Read the model definition and answer for the solid it produces. Units are mm, in the model's axes. A direction names the side the tool comes from. Round coordinates to 2 decimals unless told otherwise and drop trailing zeros. Order: outer loops, then holes, each group sorted by start corner. A loop starts at its lowest first (then second) coordinate and runs counter-clockwise, first axis right, second up. Notation, with made-up numbers: (6.5, -16) -> (37.5, -16) arc R21 cw to (37.5, -7) -> close; hole circle Ø4 at (50.5, 45). An arc over 180 degrees is marked (long way). Use a Markdown table: item, result. Add a question column.
1. Section C-C, the plane z = -10 is taken. Give the vertices of the cut face in (x, y), then the cut area to 3 significant figures.
2. Given pin 1 (1 mm diameter, centred on x = 5.5, y = -23, fed in from +Z); pin 2 (1 mm diameter, centred on x = 36.5, z = -6, fed in from -Y); pin 3 (5 mm diameter, centred on x = 19.5, y = 2, fed in from -Z), each flat-ended and moving along its own axis, determine where each tip first touches the part or whether it passes through.
3. Consider L1, parallel to Z at x = 61, y = -42.5; L2, parallel to Z at x = 25.5, y = -21.5; L3, parallel to Y at x = 32, z = -8.25. Determine where each line is inside the solid, lowest interval first. Write a range as [from, to].
4. Section D-D, the plane x = 10 is taken. Give the vertices of the cut face in (y, z).
5. For faces 1 (the face through (24.716, -15.178, -6.261)), 2 (the face through (-21.634, 16.934, 7.915)), 3 (the face through (27, -78.57, 3)), determine the directions among +Z, -Z, +X, -X, +Y, -Y from which every point of the face is accessible in a straight line to the end or side of a thin tool.
6. Section A-A, the plane x = 27 is taken. Give the vertices of the cut face in (y, z), then the cut area to 3 significant figures.
7. Section B-B, the plane y = -17 is taken. Give the vertices of the cut face in (x, z), then the cut area to 3 significant figures.
Autodesk Inventor part; units mm, degrees
ref_plane "YZ Plane" through (0, 0, 0) normal (1, 0, 0) x (0, 1, 0)
ref_plane "XZ Plane" through (0, 0, 0) normal (0, 1, 0) x (-1, 0, 0)
ref_plane "XY Plane" through (0, 0, 0) normal (0, 0, 1) x (1, 0, 0)
sketch "Sketch1" plane through (0, 0, 0) normal (0, 0, 1) x (1, 0, 0)
  line L0 (-24.4308, 23.0298) -> (77.1692, 23.0298)
  line L1 (77.1692, 23.0298) -> (77.1692, -78.5702)
  line L2 (77.1692, -78.5702) -> (-24.4308, -78.5702)
  line L3 (-24.4308, -78.5702) -> (-24.4308, 23.0298)
  point P0 (0, 0)
  dimension "d0" = 101.6
  dimension "d1" = 101.6
extrude "Extrusion1" add sketch "Sketch1" along normal blind 6.35
sketch "Sketch2" plane through (0, 0, 6.35) normal (0, 0, 1) x (1, 0, 0)
  line L0 (-24.4308, 23.0298) -> (26.3692, 23.0298)
  line L1 (26.3692, 23.0298) -> (26.3692, -27.7702)
  line L2 (26.3692, -27.7702) -> (-24.4308, -27.7702)
  line L3 (-24.4308, -27.7702) -> (-24.4308, 23.0298)
  circle A0 centre (26.3692, -27.7702) radius 12.7
  point P0 (0, 0)
  dimension "d4" = 50.8
  dimension "d5" = 50.8
  dimension "d6" = 25.4
extrude "Extrusion2" cut sketch "Sketch2" against normal blind 6.35 contours A0 L2 L1 | L1 L2 A0
sketch "Sketch3" plane through (0, 0, 6.35) normal (0, 0, 1) x (1, 0, 0)
  line L0 (-24.4308, 23.0298) -> (77.1692, 23.0298)
  line L1 (-24.4308, -78.5702) -> (-24.4308, 23.0298)
  line L2 (-24.4308, 23.0298) -> (-24.4308, -27.7702)
  line L3 (-24.4308, -27.7702) -> (-24.4308, 11.9935)
  line L4 (-24.4308, 11.9935) -> (-13.3818, 11.9935)
  line L5 (-13.3818, 11.9935) -> (-13.3818, 23.0298)
  line L6 (-13.3818, 23.0298) -> (-24.4308, 23.0298)
  line L7 (-24.4308, 23.0298) -> (-24.4308, 11.9935)
  circle A0 centre (-13.3818, 11.9935) radius 3.175
  point P0 (0, 0)
  dimension "d9" = 50.8
  dimension "d10" = 39.7637
  dimension "d11" = 11.049
  dimension "d12" = 6.35
extrude "Extrusion3" add sketch "Sketch3" along normal blind 6.35 contours A0 L4 L5 | L5 L4 A0
sketch "Sketch4" plane through (0, 0, 6.35) normal (0, 0, 1) x (1, 0, 0)
  circle A0 centre (26.3692, -27.7702) radius 12.7
  point P0 (0, 0)
extrude "Extrusion4" add sketch "Sketch4" against normal blind 19.05
sketch "Sketch5" plane through (0, 0, 6.35) normal (0, 0, 1) x (1, 0, 0)
  line L0 (-24.4308, -78.5702) -> (-24.4308, 23.0298)
  line L1 (-24.4308, 23.0298) -> (-24.4308, -27.7702)
  line L2 (-24.4308, -27.7702) -> (-24.4308, 17.0735)
  line L3 (-24.4308, 23.0298) -> (-18.4618, 23.0298)
  line L4 (-18.4618, 23.0298) -> (-18.4618, 17.0735)
  line L5 (-18.4618, 17.0735) -> (-24.4308, 17.0735)
  line L6 (-24.4308, 17.0735) -> (-24.4308, 23.0298)
  circle A0 centre (-18.4618, 17.0735) radius 3.175
  point P0 (0, 0)
  dimension "d17" = 50.8
  dimension "d18" = 44.8437
  dimension "d19" = 5.969
  dimension "d20" = 6.35
extrude "Extrusion5" add sketch "Sketch5" along normal blind 3.175 contours A0 L4 L5 | L5 L4 A0
sketch "Sketch6" plane through (-13.3818, 11.9935, 12.7) normal (0, 0, 1) x (1, 0, 0)
  circle A0 centre (0, 0) radius 3.175
  point P0 (13.3818, -11.9935)
extrude "Extrusion6" cut sketch "Sketch6" against normal blind 6.35
properties part number "lasiness"
Verdict:
| question | item | result |
|---|---|---|
| 1 | outline | circle Ø25.4 at (26.37, -27.77) |
| 1 | area | 507 mm2 |
| 2 | pin 1 | stops at z = 6.35 |
| 2 | pin 2 | stops at y = -36.05 |
| 2 | pin 3 | stops at z = 0 |
| 3 | L1 | z = [0, 6.35] |
| 3 | L2 | z = [-12.7, 6.35] |
| 3 | L3 | y = [-39.15, -16.39] |
| 4 | outline | (-78.57, 0) -> (23.03, 0) -> (23.03, 6.35) -> (-78.57, 6.35) -> close |
| 5 | face 1 | -Z |
| 5 | face 2 | +Z |
| 5 | face 3 | +Z, -Z, +X, -X, -Y |
| 6 | outline | (-78.57, 0) -> (-40.45, 0) -> (-40.45, -12.7) -> (-15.09, -12.7) -> (-15.09, 0) -> (23.03, 0) -> (23.03, 6.35) -> (-78.57, 6.35) -> close |
| 6 | area | 967 mm2 |
| 7 | outline | (-24.43, 0) -> (19.64, 0) -> (19.64, -12.7) -> (33.1, -12.7) -> (33.1, 0) -> (77.17, 0) -> (77.17, 6.35) -> (-24.43, 6.35) -> close |
| 7 | area | 816 mm2 |
